Autodesk Inventor part; units mm, degrees
ref_plane "YZ Plane" through (0, 0, 0) normal (1, 0, 0) x (0, 1, 0)
ref_plane "XZ Plane" through (0, 0, 0) normal (0, 1, 0) x (-1, 0, 0)
ref_plane "XY Plane" through (0, 0, 0) normal (0, 0, 1) x (1, 0, 0)
ref_plane "Arbeitsebene1" through (0, 0, 0) normal (0, 0, 1) x (1, 0, 0)
sketch "Skizze1" plane through (0, 0, 0) normal (0, 0, 1) x (1, 0, 0)
  circle A0 centre (-27.8589, -14.9953) radius 1.4
  circle A1 centre (-27.8589, -39.949) radius 1.4
  line L0 (-21.8589, -42.949) -> (-33.8589, -42.949)
  line L1 (-33.8589, -42.949) -> (-33.8589, -11.9953)
  line L2 (-33.8589, -11.9953) -> (-21.8589, -11.9953)
  line L3 (-21.8589, -11.9953) -> (-21.8589, -42.949)
  line L4 (-21.8589, -42.949) -> (-33.8589, -11.9953) construction
  line L5 (-33.8589, -42.949) -> (-21.8589, -11.9953) construction
  line L6 (-59.9, -42.75) -> (59.9, -42.75)
  point P0 (0, 0)
  point P1 (-27.8589, -27.4722)
  point P2 (-33.8589, -42.75)
  point P3 (-21.8589, -42.75)
  dimension "d0" = 24.9538
  dimension "d1" = 3
  dimension "d2" = 3
  dimension "d3" = 12
extrude "Extrusion1" add sketch "Skizze1" along normal blind 4 contours L6 L1 L2 L3
fillet "Rundung1" radius 2 4 edges at (-21.8589, -11.9953, 2) (-33.8589, -11.9953, 2) (-21.8589, -42.75, 2) (-33.8589, -42.75, 2)
sketch "Skizze2" plane through (-21.8589, -40.75, 0) normal (1, 0, 0) x (0, 0, -1)
  circle A0 centre (4.8526, 13) radius 4.7625
  circle A1 centre (4.3786, 13) radius 5.5
  point P0 (0, 40.75)
  dimension "d7" = 11
extrude "Extrusion2" cut sketch "Skizze2" against normal through all contours A0 | A1
properties part number "20_M12_Lens_Fixation_1"
Geometry check sheet. Reference: the model listing, model coordinates, mm. Give positions to 0.01 mm unless a question says otherwise; leave off trailing zeros. Loops run counter-clockwise (first coordinate to the right, second up) from the corner with the lowest first, then second, coordinate; pieces in that order, holes last. Notation, with made-up numbers: M -17.5,-9.5 L 9.5,-9.5 A18 ccw 9.5,-3.5 Z; hole C -38.5,-13.75 d9. An arc over 180 degrees is marked long. Write item = value, one per line. Start each with the question number.
1. Section check A-A, the plane y = -16. Enter the section's corners in (x, z).
2. Section check B-B, the plane x = -28. Enter the section's corners in (y, z), plus the area to 3 significant figures.
3. Thickness scan on probe 1 along Y at (x, z) = (-29, 1.65); probe 2 along X at (y, z) = (-15, 2.15); probe 3 along Y at (x, z) = (-32, 2.6). Record the ranges inside material, lowest first.
4. Draft check along X on faces 1 (the face through (-33.289, -42.149, 2.028)), 2 (the face through (-27.21, -38.71, 1.97)), 3 (the face through (-22.46, -42.18, 2.03)), 4 (the face through (-28, -37, 0)). Enter one of: +X half, -X half, draft (parallel to the pull), parting line (faces both ways), or undercut.
5. Section check D-D, the plane z = 1.5. Enter the section's corners in (x, y).
6. Section check C-C, the plane x = -31.25. Enter the section's corners in (y, z).
Values follow:
q1.outline = M -33.86,0 L -28.83,0 L -28.83,4 L -33.86,4 Z; M -26.88,0 L -21.86,0 L -21.86,4 L -26.88,4 Z
q2.outline = M -42.75,0 L -41.34,0 L -41.34,4 L -42.75,4 Z; M -38.56,0 L -31.08,0 A5.5 cw -24.42,0 L -16.39,0 L -16.39,4 L -38.56,4 Z; M -13.6,0 L -12,0 L -12,4 L -13.6,4 Z
q2.area = 95.6 mm^2
q3.probe_1 = -42.75 to -40.76, -39.14 to -15.81, -14.18 to -12
q3.probe_2 = -33.86 to -29.26, -26.46 to -21.86
q3.probe_3 = -42.75 to -12
q4.face_1 = -X half
q4.face_2 = undercut
q4.face_3 = +X half
q4.face_4 = draft
q5.outline = M -33.86,-40.75 A2 ccw -31.86,-42.75 L -23.86,-42.75 A2 ccw -21.86,-40.75 L -21.86,-14 A2 ccw -23.86,-12 L -31.86,-12 A2 ccw -33.86,-14 Z; hole C -27.86,-39.95 d2.8; hole C -27.86,-15 d2.8
q6.outline = M -42.75,0 L -31.08,0 A5.5 cw -24.42,0 L -12,0 L -12,4 L -42.75,4 Z
